Part model, mm, in its own coordinate system. Face numbers are marked on the shaded views. A direction names the side the tool comes from. Round coordinates to 2 decimals unless told otherwise and drop trailing zeros. Loops run counter-clockwise (first coordinate to the right, second up) from the corner with the lowest first, then second, coordinate; pieces in that order, holes last.
(1) Cut at B-B on y = 30. List the corners of the cut face in (x, z).
(2) Cut at C-C on y = 24.5. List the corners of the cut face in (x, z).
(3) Mould opens along X. For the marked faces 1 and 2 say: +X half, -X half, draft (parallel to the pull), parting line (faces both ways), or undercut.
(4) Cut at A-A on x = 0. List the corners of the cut face in (y, z).
(5) Flat gauge pins, fed straight in: pin 1 (5 mm diameter, centred on y = 33, z = 2.5, fed in from -X); pin 2 (4 mm diameter, centred on x = 0, z = 0, fed in from -Y); pin 3 (1 mm diameter, centred on y = 25.5, z = -2.5, fed in from -X); pin 4 (1 mm diameter, centred on x = -1, y = 17, fed in from -Z). Where does each tip first touch, or does it go through?
(6) Probe probe 1 along X at (y, z) = (32, 0); probe 2 along Z at (x, y) = (0, 17.75). List the from-to ranges inside material, lowest first.
(7) Tool access for the marked faces 3, 4 and 5: list every direction of +Z, -Z, +X, -X, +Y, -Y with a clear straight run to the whole face (end or side of a thin tool).
Autodesk Inventor part; units mm, degrees
ref_plane "Work Plane3" through (0, 10, 0) normal (0, 1, 0) x (1, 0, 0)
ref_plane "Work Plane1" through (0, 11.25, 0) normal (0, 1, 0) x (1, 0, 0)
ref_plane "Work Plane2" through (0, 26.5, 0) normal (0, 1, 0) x (1, 0, 0)
ref_plane "Work Plane3" through (0, 10, 0) normal (0, 1, 0) x (1, 0, 0)
sketch "Sketch2" plane through (0, 10, 0) normal (0, 1, 0) x (1, 0, 0)
  circle A0 centre (0, 0) radius 4
  circle A1 centre (0, 0) radius 4.25
  dimension "d4" = 8
  dimension "d5" = 0.25
extrude "Extrusion2" add sketch "Sketch2" along normal blind 15
extrude "Extrusion3" cut sketch "Sketch2" along normal blind 2.5
ref_plane "Work Plane1" through (0, 11.25, 0) normal (0, 1, 0) x (1, 0, 0)
ref_plane "Work Plane2" through (0, 26.5, 0) normal (0, 1, 0) x (1, 0, 0)
sketch "Sketch6" plane through (0, 26.5, 0) normal (0, 1, 0) x (1, 0, 0)
  circle A0 centre (0, 0) radius 2.75
  dimension "d17" = 5.5
loft "Loft1" add profiles "Sketch6" section 1 edges at (-4.25, 25, 0)
sketch "Sketch7" plane through (0, 26.5, 0) normal (0, 1, 0) x (1, 0, 0)
  circle A0 centre (0, 0) radius 2.5
  dimension "d22" = 5
extrude "Extrusion4" cut sketch "Sketch7" against normal blind 2.5
sketch "Sketch8" plane through (0, 26.5, 0) normal (0, 1, 0) x (1, 0, 0)
  circle A0 centre (0, 0) radius 2.75
  circle A1 centre (0, 0) radius 2.5
  dimension "d25" = 5.5
  dimension "d26" = 0.25
extrude "Extrusion5" add sketch "Sketch8" along normal blind 10
properties part number "5mm to 8mm holder" material "PET Plastic"
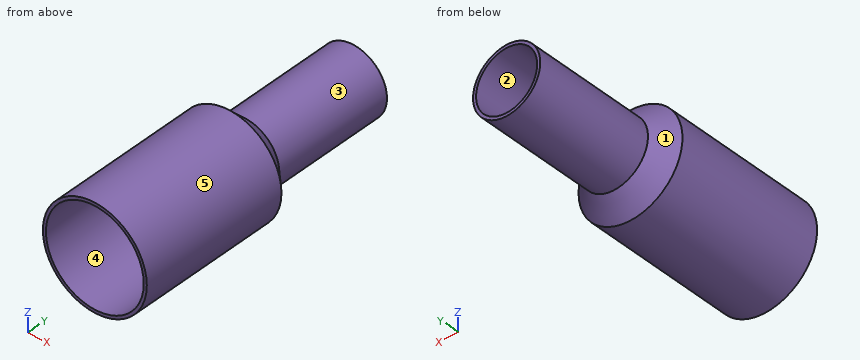
Final values:
1. outline: circle Ø5.5 at (0, 0); hole circle Ø5 at (0, 0)
2. outline: circle Ø8.5 at (0, 0); hole circle Ø8 at (0, 0)
3. face 1: parting line
3. face 2: undercut
4. outline: (12.5, -4.25) - (25, -4.25) - (26.5, -2.75) - (36.5, -2.75) - (36.5, -2.5) - (25, -2.5) - (25, -4) - (12.5, -4) - close; (12.5, 4) - (25, 4) - (25, 2.5) - (36.5, 2.5) - (36.5, 2.75) - (26.5, 2.75) - (25, 4.25) - (12.5, 4.25) - close
5. pin 1: stops at x = -2.75
5. pin 2: passes through
5. pin 3: stops at x = -3.53
5. pin 4: stops at z = -4.22
6. probe 1: x = -2.75 to -2.5, 2.5 to 2.75
6. probe 2: z = -4.25 to -4, 4 to 4.25
7. face 3: +Y
7. face 4: -Y
7. face 5: +Y, -Y
